The drawing under review shows one solid part. Ordinate dimensions are in mm from its lowest x, y, z. Coordinates: 2 decimals unless noted, no trailing zeros. Order: outer loops, then holes, each group sorted by start corner. A loop starts at its lowest first (then second) coordinate and runs counter-clockwise, first axis right, second up.
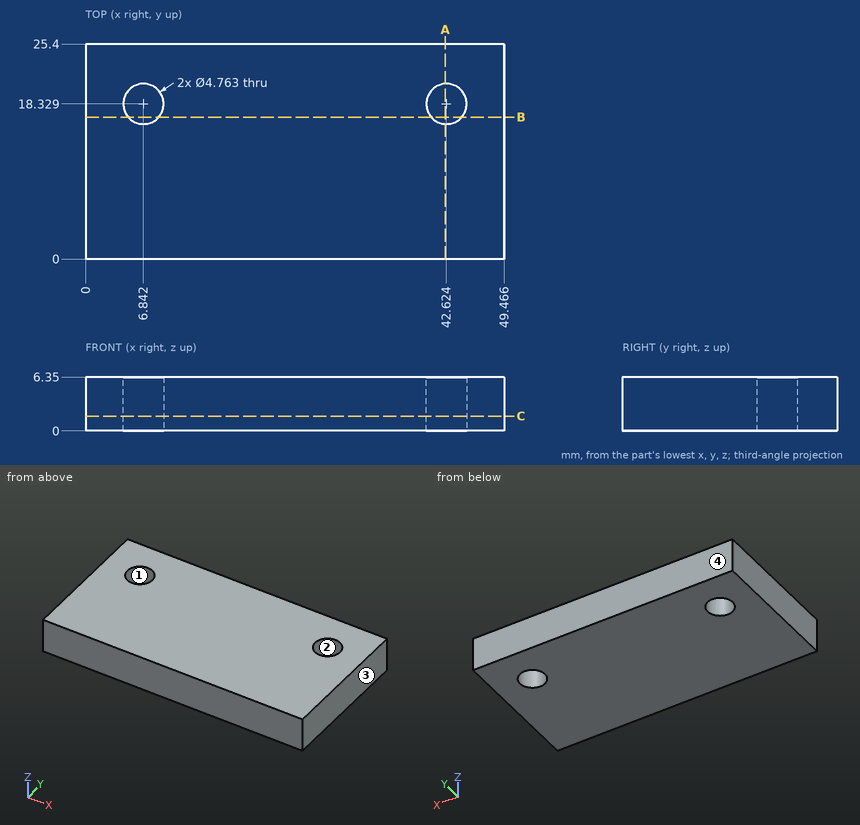
1. Add section C-C (z = 1.75). Give the boundary of the cut face in (x, y) (1 decimal), and give its area (3 significant figures).
2. Add section A-A (x = 42.5). Give the boundary of the cut face in (y, z), and give its area (3 significant figures).
3. To check wall thickness, follow line 1 (X direction, y = 19, z = 3.25) (1 decimal); line 2 (X direction, y = 20, z = 4.5) (1 decimal); line 3 (Y direction, x = 7.5, z = 1). State the ranges of each line that lie inside material, in increasing order.
4. Mouldability with a two-part tool opening along Y and no side actions: class the marked faces 1, 2, 3 and 4 as pulls with the +Y half, pulls with the -Y half, needs draft (parallel to the pull), parting line crosses it, or undercut.
5. Insertion check: pin 1 (4.5 mm diameter, centred on x = 6.84, y = 18.33, fed in from +Z). The pin has a flat end and moves straight along its axis. Give the tip position at first contact, or say it passes through.
6. Add section B-B (y = 16.75). State how many separate pieces and enclosed holes the cut face has, and give its area (3 significant figures).
Solution:
1. outline: (0, 0) - (49.5, 0) - (49.5, 25.4) - (0, 25.4) - close; hole circle Ø4.8 at (6.8, 18.3); hole circle Ø4.8 at (42.6, 18.3)
1. area: 1,220 mm2
2. outline: (0, 0) - (15.95, 0) - (15.95, 6.35) - (0, 6.35) - close; (20.71, 0) - (25.4, 0) - (25.4, 6.35) - (20.71, 6.35) - close
2. area: 131 mm2
3. line 1: x = 0 to 4.6, 9.1 to 40.3, 44.9 to 49.5
3. line 2: x = 0 to 5.1, 8.5 to 40.9, 44.3 to 49.5
3. line 3: y = 0 to 16.04, 20.62 to 25.4
4. face 1: undercut
4. face 2: undercut
4. face 3: needs draft
4. face 4: pulls with the +Y half
5. pin 1: passes through
6. separate pieces: 3
6. enclosed holes: 0
6. area: 269 mm2
